Verification items for the finished model (mm, model axes). Face numbers are marked on the shaded views. A direction names the side the tool comes from. Round coordinates to 2 decimals unless told otherwise and drop trailing zeros. Order: outer loops, then holes, each group sorted by start corner. A loop starts at its lowest first (then second) coordinate and runs counter-clockwise, first axis right, second up. Notation, with made-up numbers: (8.5, 71) -> (67.5, 71) arc R22 ccw to (67.5, 91) -> close; hole circle Ø8 at (4, 48). An arc over 180 degrees is marked (long way). Put each result on its own line as item: value.
from build123d import *

# Parameters (mm, degrees)
SCHIZZO1_R                         = 110.5
SCHIZZO1_R_2                       = 103
ESTRUSIONE_ESTRUSIONE1_DEPTH       = 136.9
ESTRUSIONE_ESTRUSIONE2_DEPTH       = 10
ESTRUSIONE_ESTRUSIONE2_DEPTH_BACK  = 20
SCHIZZO1_3_R                       = 103
SCHIZZO1_3_R_2                     = 95
SMUSSO1_SIZE                       = 10
SMUSSO2_SIZE                       = 2
SCHIZZO2_R                         = 110.5
SCHIZZO2_R_2                       = 97.5
ESTRUSIONE_ESTRUSIONE3_DEPTH       = 8.1
SMUSSO3_SIZE                       = 5.5
FORO_PER_VITE_M4_1_D               = 5.6
FORO_PER_VITE_M4_1_DEPTH           = 8.1
FORO_PER_VITE_M4_1_TIP             = 1.682409733
FORO_PER_VITE_M4_2_D               = 5.6
FORO_PER_VITE_M4_2_DEPTH           = 8.1
FORO_PER_VITE_M4_2_TIP             = 1.682409733
FORO_PER_VITE_M4_2_ON_FACE_2_D     = 5.6
FORO_PER_VITE_M4_2_ON_FACE_2_DEPTH = 8.1
FORO_PER_VITE_M4_2_ON_FACE_2_TIP   = 1.682409733
FORO_PER_VITE_M4_2_ON_FACE_3_D     = 5.6
FORO_PER_VITE_M4_2_ON_FACE_3_DEPTH = 8.1
FORO_PER_VITE_M4_2_ON_FACE_3_TIP   = 1.682409733
FORO_PER_VITE_M4_2_ON_FACE_4_D     = 5.6
FORO_PER_VITE_M4_2_ON_FACE_4_DEPTH = 8.1
FORO_PER_VITE_M4_2_ON_FACE_4_TIP   = 1.682409733
ESTRUSIONE_ESTRUSIONE4_DEPTH       = 46
SMUSSO4_SIZE                       = 2


# Read off the part's stored shape, not the designer's step: Foro per Vite M4-3
# Some blends are built 0.0001 mm under size
with BuildPart() as part:
    # Schizzo1 → Estrusione-Estrusione1 (new body)
    with BuildSketch(Plane(origin=(0, 0, 0), x_dir=(1, 0, 0), z_dir=(0, 1, 0))):
        with Locations(Location((0, 0, 0), (0, 0, 270))):
            Circle(SCHIZZO1_R)
        with Locations(Location((0, 0, 0), (0, 0, 270))):
            Circle(SCHIZZO1_R_2, mode=Mode.SUBTRACT)
    extrude(amount=ESTRUSIONE_ESTRUSIONE1_DEPTH)

    # Schizzo1<3> → Estrusione-Estrusione2 (add, two sides: drawn at the far end of the back side and taken through both)
    with BuildSketch(Plane(origin=(0, 0, 0), x_dir=(1, 0, 0), z_dir=(0, 1, 0)).offset(-ESTRUSIONE_ESTRUSIONE2_DEPTH_BACK)):
        with Locations(Location((0, 0, 0), (0, 0, 270))):
            Circle(SCHIZZO1_3_R)
        with Locations(Location((0, 0, 0), (0, 0, 270))):
            Circle(SCHIZZO1_3_R_2, mode=Mode.SUBTRACT)
    extrude(amount=ESTRUSIONE_ESTRUSIONE2_DEPTH + ESTRUSIONE_ESTRUSIONE2_DEPTH_BACK)

    # Smusso1
    # the kernel refuses this chamfer: 10 mm, written as the material it takes off along each edge
    with BuildSketch(Plane(origin=(0, 10, 0), x_dir=(0, 0, 1), z_dir=(-1, 0, 0))) as smusso1_piece_1_section:
        Polygon((95 + SMUSSO1_SIZE, 0), (95, -SMUSSO1_SIZE), (95, 0), align=None)
    smusso1_piece_1 = revolve(axis=Axis((0, 10, 0), (0, 1, 0)), mode=Mode.PRIVATE)
    smusso1_piece_1 = smusso1_piece_1 & Plane(origin=(0, 4.08333284, 0), x_dir=(0, 0, 1), z_dir=(0, -1, 0)) * Cylinder(103, 420, mode=Mode.PRIVATE)
    add(smusso1_piece_1, mode=Mode.SUBTRACT)

    # Smusso2
    smusso2_edges = [part.edges().sort_by_distance(p)[0] for p in [
        (0, -20, -95),
        (0, -20, -103),
    ]]
    chamfer(smusso2_edges, length=SMUSSO2_SIZE)

    # Schizzo2 → Estrusione-Estrusione3 (add)
    with BuildSketch(Plane(origin=(0, 136.9, 0), x_dir=(1, 0, 0), z_dir=(0, 1, 0))):
        with Locations(Location((0, 0, 0), (0, 0, 270))):
            Circle(SCHIZZO2_R)
        with Locations(Location((0, 0, 0), (0, 0, 270))):
            Circle(SCHIZZO2_R_2, mode=Mode.SUBTRACT)
    extrude(amount=ESTRUSIONE_ESTRUSIONE3_DEPTH)

    # Smusso3
    smusso3_edges = [part.edges().sort_by_distance(p)[0] for p in [
        (0, 136.9, -103),
    ]]
    chamfer(smusso3_edges, length=SMUSSO3_SIZE - 0.0001)  # a hair under: the kernel refuses the full size

    # Foro per Vite M4-1
    with Locations(Plane(origin=(0, 145, 0), x_dir=(1, 0, 0), z_dir=(0, 1, 0))):
        with Locations((0, 103), (0, -103), (103, 0), (-103, 0)):
            Hole(FORO_PER_VITE_M4_1_D / 2, depth=FORO_PER_VITE_M4_1_DEPTH)
            with Locations((0, 0, -(FORO_PER_VITE_M4_1_DEPTH + FORO_PER_VITE_M4_1_TIP / 2))):  # 118° drill point
                Cone(0, FORO_PER_VITE_M4_1_D / 2, FORO_PER_VITE_M4_1_TIP, mode=Mode.SUBTRACT)

    # Foro per Vite M4-2
    with Locations(Plane(origin=(72.831998462, -10, -72.831998462), x_dir=(0.707106781187, 0, 0.707106781187), z_dir=(0.707106781187, 0, -0.707106781187))):
        with Locations((0, 0)):
            Hole(FORO_PER_VITE_M4_2_D / 2, depth=FORO_PER_VITE_M4_2_DEPTH)
            with Locations((0, 0, -(FORO_PER_VITE_M4_2_DEPTH + FORO_PER_VITE_M4_2_TIP / 2))):  # 118° drill point
                Cone(0, FORO_PER_VITE_M4_2_D / 2, FORO_PER_VITE_M4_2_TIP, mode=Mode.SUBTRACT)

    # Foro per Vite M4-2 on face 2
    with Locations(Plane(origin=(-72.831998462, -10, -72.831998462), x_dir=(-0.707106781187, 0, 0.707106781187), z_dir=(-0.707106781187, 0, -0.707106781187))):
        with Locations((0, 0)):
            Hole(FORO_PER_VITE_M4_2_ON_FACE_2_D / 2, depth=FORO_PER_VITE_M4_2_ON_FACE_2_DEPTH)
            with Locations((0, 0, -(FORO_PER_VITE_M4_2_ON_FACE_2_DEPTH + FORO_PER_VITE_M4_2_ON_FACE_2_TIP / 2))):  # 118° drill point
                Cone(0, FORO_PER_VITE_M4_2_ON_FACE_2_D / 2, FORO_PER_VITE_M4_2_ON_FACE_2_TIP, mode=Mode.SUBTRACT)

    # Foro per Vite M4-2 on face 3
    with Locations(Plane(origin=(-72.831998462, -10, 72.831998462), x_dir=(0.707106781187, 0, 0.707106781187), z_dir=(-0.707106781187, 0, 0.707106781187))):
        with Locations((0, 0)):
            Hole(FORO_PER_VITE_M4_2_ON_FACE_3_D / 2, depth=FORO_PER_VITE_M4_2_ON_FACE_3_DEPTH)
            with Locations((0, 0, -(FORO_PER_VITE_M4_2_ON_FACE_3_DEPTH + FORO_PER_VITE_M4_2_ON_FACE_3_TIP / 2))):  # 118° drill point
                Cone(0, FORO_PER_VITE_M4_2_ON_FACE_3_D / 2, FORO_PER_VITE_M4_2_ON_FACE_3_TIP, mode=Mode.SUBTRACT)

    # Foro per Vite M4-2 on face 4
    with Locations(Plane(origin=(72.831998462, -10, 72.831998462), x_dir=(0.707106781187, 0, -0.707106781187), z_dir=(0.707106781187, 0, 0.707106781187))):
        with Locations((0, 0)):
            Hole(FORO_PER_VITE_M4_2_ON_FACE_4_D / 2, depth=FORO_PER_VITE_M4_2_ON_FACE_4_DEPTH)
            with Locations((0, 0, -(FORO_PER_VITE_M4_2_ON_FACE_4_DEPTH + FORO_PER_VITE_M4_2_ON_FACE_4_TIP / 2))):  # 118° drill point
                Cone(0, FORO_PER_VITE_M4_2_ON_FACE_4_D / 2, FORO_PER_VITE_M4_2_ON_FACE_4_TIP, mode=Mode.SUBTRACT)

    # Schizzo7 → Estrusione-Estrusione4 (add)
    with BuildSketch(Plane.XZ.offset(-30)):
        with BuildLine():
            Line((-35, -104.810543363), (-35, -110.5))
            Line((-35, -110.5), (-35, -112.5))
            Line((-35, -112.5), (35, -112.5))
            Line((35, -112.5), (35, -110.5))
            Line((35, -110.5), (35, -104.810543363))
            ThreePointArc((35, -104.810543363), (0, -110.5), (-35, -104.810543363))
        make_face()
    extrude(amount=-ESTRUSIONE_ESTRUSIONE4_DEPTH)

    # Smusso4
    smusso4_edges = [part.edges().sort_by_distance(p)[0] for p in [
        (0, 76, -110.5),
        (0, 30, -110.5),
    ]]
    chamfer(smusso4_edges, length=SMUSSO4_SIZE - 0.0001)  # a hair under: the kernel refuses the full size

    # Foro per Vite M4-3 outline → Foro per Vite M4-3 (revolve, cut)
    with BuildSketch(Plane(origin=(-29, 36, 0), x_dir=(1, 0, 0), z_dir=(0, -1, 0))):
        Polygon((2.7, -104.4), (0, -102.777676329), (0, -112.5), (2.7, -112.5), align=None)
    revolve(axis=Axis((-29, 36, 0), (0, 0, 1)), mode=Mode.SUBTRACT)

    # Foro per Vite M4-3 2 outline → Foro per Vite M4-3 2 (revolve, cut)
    with BuildSketch(Plane(origin=(29, 70, 0), x_dir=(1, 0, 0), z_dir=(0, -1, 0))):
        Polygon((2.7, -104.4), (0, -102.777676329), (0, -112.5), (2.7, -112.5), align=None)
    revolve(axis=Axis((29, 70, 0), (0, 0, 1)), mode=Mode.SUBTRACT)

    # Foro per Vite M4-3 3 outline → Foro per Vite M4-3 3 (revolve, cut)
    with BuildSketch(Plane(origin=(-29, 70, 0), x_dir=(1, 0, 0), z_dir=(0, -1, 0))):
        Polygon((2.7, -104.4), (0, -102.777676329), (0, -112.5), (2.7, -112.5), align=None)
    revolve(axis=Axis((-29, 70, 0), (0, 0, 1)), mode=Mode.SUBTRACT)

    # Foro per Vite M4-3 4 outline → Foro per Vite M4-3 4 (revolve, cut)
    with BuildSketch(Plane(origin=(29, 36, 0), x_dir=(1, 0, 0), z_dir=(0, -1, 0))):
        Polygon((2.7, -104.4), (0, -102.777676329), (0, -112.5), (2.7, -112.5), align=None)
    revolve(axis=Axis((29, 36, 0), (0, 0, 1)), mode=Mode.SUBTRACT)


solid = part.part
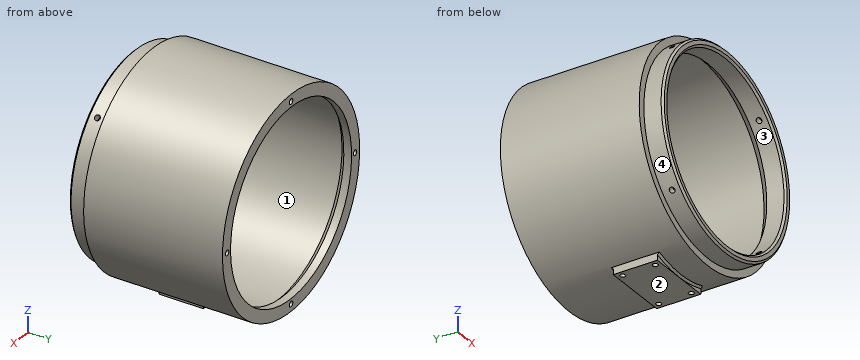
Item 1: Section check A-A on y = 5. Record the boundary of the cut face in (x, z), then the cut area to 3 significant figures.
Check sheet entries:
outline: circle Ø221 at (0, 0); hole circle Ø200 at (0, 0)
area: 6,940 mm^2
Item 2: Release check for a two-part mould opening along Y. For the marked faces 1 and 2 record: +Y half, -Y half, draft (parallel to the pull), parting line (faces both ways), or undercut.
Check sheet entries:
face 1: undercut
face 2: draft
Item 3: Gauge pin test, flat ends, axial feed: pin 1 Ø4.5 at (x, z) = (-103, 0) entering from +Y; pin 2 Ø2 at (y, z) = (122, 80) entering from -X; pin 3 Ø7 at (x, y) = (-29, 70) entering from +Z. Record the tip position at first contact, or that the pin passes through.
Check sheet entries:
pin 1: stops at y = 136.57
pin 2: stops at x = -77.26
pin 3: stops at z = 107.52
Item 4: Tool access check on the marked faces 3 and 4. Record the directions out of +Z, -Z, +X, -X, +Y, -Y that give a thin tool (end or side, any length) a straight path to the whole face; none if there is none.
Check sheet entries:
face 3: +Y, -Y
face 4: -Y
Item 5: Material ranges on L1, parallel to Y at x = 29, z = -109.75; L2, parallel to Y at x = -29, z = -105.75; L3, parallel to Z at x = -80, y = 32 (3 decimals), recorded low to high. Write a range as [from, to].
Check sheet entries:
L1: y = [30, 33.3], [38.7, 67.3], [72.7, 76]
L2: y = [0, 33.3], [38.7, 67.3], [72.7, 145]
L3: z = [-76.225, -64.877], [64.877, 76.225]
